Input: part model. Units: mm. Frame: model coordinates. Coordinates: 2 decimals unless noted, no trailing zeros. Write each loop counter-clockwise with the first axis right and the second up, starting at its lowest first coordinate (ties: lowest second). Pieces come first, ordered by that corner, then holes. Notation, with made-up numbers: M 66.25,72.5 L 99.25,72.5 A6 ccw 99.25,82.5 Z; hole C 21,44 d7. An arc over 180 degrees is marked long. Answer as a JSON object with one key per item and string values. Group by question number.
from build123d import *

# Parameters (mm, degrees)
SKETCH1_R              = 3.175
SKETCH1_R_2            = 1.99644
BOSS_EXTRUDE1_DEPTH    = 12.7
CUT_EXTRUDE1_START     = -3.175
CUT_EXTRUDE1_OUTLINE_R = 2.54
CUT_EXTRUDE1_DEPTH     = 3.175


# Read off the part's stored shape, not the designer's step: Cut-Extrude1
with BuildPart() as part:
    # Sketch1 → Boss-Extrude1 (new body)
    with BuildSketch(Plane(origin=(0, 0, 0), x_dir=(1, 0, 0), z_dir=(0, 1, 0))):
        with Locations(Location((0, 0, 0), (0, 0, 90))):
            Circle(SKETCH1_R)
        with Locations(Location((0, 0, 0), (0, 0, 90))):
            Circle(SKETCH1_R_2, mode=Mode.SUBTRACT)
    extrude(amount=BOSS_EXTRUDE1_DEPTH)

    # Cut-Extrude1 outline → Cut-Extrude1 (cut)
    with BuildSketch(Plane(origin=(0, 12.7, -3.175), x_dir=(-1, 0, 0), z_dir=(0, 0, -1)).offset(CUT_EXTRUDE1_START)):
        with Locations((0, -3.68808)):
            Circle(CUT_EXTRUDE1_OUTLINE_R)
    extrude(amount=CUT_EXTRUDE1_DEPTH, mode=Mode.SUBTRACT)


solid = part.part
Q1. Line query: line 1 (X direction, y = 2.75, z = 0) (3 decimals); line 2 (X direction, y = 12.25, z = -0.5); line 3 (Y direction, x = -1, z = -2). Output: solid intervals per line, ascending. Write a range as from..to.
Q2. Draft query along Y for faces 1 (the flat face through (2, 12.7, -1)), 2 (the cylindrical face through (2.02, 7.47, -1.57)), 3 (the flat face through (2, 0, -1)). Return one class per face: released by +Y, released by -Y, zero draft, split by the parting line, or undercut.
Q3. Section B-B, the plane z = -1.5. Return the cut outline in (x, y).
Q4. Section D-D, the plane z = 0.5. Return the cut outline in (x, y), and give its area (3 significant figures).
Q5. Section A-A, the plane x = 0. Return the cut outline in (y, z) (3 decimals).
Q6. Section C-C, the plane y = 5.5. Return the cut outline in (x, z) (3 decimals).
Q7. Pin query (flat end, axial travel): pin 1 Ø1 at (y, z) = (5.5, 1.5) entering from -X; pin 2 Ø2.5 at (x, z) = (0, 0) entering from +Y. Return the tip coordinate at first contact, or that it passes through.
Filled in:
{
 "1": {"line 1": "-3.175..-1.996, 1.996..3.175", "line 2": "-3.14..-1.93, 1.93..3.14", "line 3": "0..6.68, 11.35..12.7"},
 "2": {"face 1": "released by +Y", "face 2": "undercut", "face 3": "released by -Y"},
 "3": {"outline": "M -2.8,0 L -1.32,0 L -1.32,6.84 A2.54 cw -1.32,11.18 L -1.32,12.7 L -2.8,12.7 Z; M 1.32,0 L 2.8,0 L 2.8,12.7 L 1.32,12.7 L 1.32,11.18 A2.54 cw 1.32,6.84 Z"},
 "4": {"outline": "M -3.14,0 L -1.93,0 L -1.93,12.7 L -3.14,12.7 Z; M 1.93,0 L 3.14,0 L 3.14,12.7 L 1.93,12.7 Z", "area": "30.5 mm^2"},
 "5": {"outline": "M 0,-3.175 L 6.472,-3.175 L 6.472,-1.996 L 0,-1.996 Z; M 0,1.996 L 12.7,1.996 L 12.7,3.175 L 0,3.175 Z; M 11.552,-3.175 L 12.7,-3.175 L 12.7,-1.996 L 11.552,-1.996 Z"},
 "6": {"outline": "C 0,0 d6.35; hole C 0,0 d3.993"},
 "7": {"pin 1": "x = -3.01", "pin 2": "through"}
}
